from build123d import *

# Parameters (mm, degrees)
SKETCH2_W           = 110
SKETCH2_H           = 83
SKETCH2_W_2         = 10
SKETCH2_H_2         = 40
BOSS_EXTRUDE1_DEPTH = 9
SKETCH4_W           = 103
SKETCH4_H           = 77.5
CUT_EXTRUDE1_DEPTH  = 6


with BuildPart() as part:
    # Sketch2 → Boss-Extrude1 (new body)
    with BuildSketch(Plane(origin=(0, 0, 0), x_dir=(1, 0, 0), z_dir=(0, 1, 0))):
        Rectangle(SKETCH2_W, SKETCH2_H)
        with Locations((46, 0)):
            Rectangle(SKETCH2_W_2, SKETCH2_H_2, mode=Mode.SUBTRACT)
    extrude(amount=BOSS_EXTRUDE1_DEPTH)

    # Sketch4 → Cut-Extrude1 (cut)
    with BuildSketch(Plane(origin=(0, 9, 0), x_dir=(1, 0, 0), z_dir=(0, 1, 0))):
        Rectangle(SKETCH4_W, SKETCH4_H)
    extrude(amount=-CUT_EXTRUDE1_DEPTH, mode=Mode.SUBTRACT)


solid = part.part
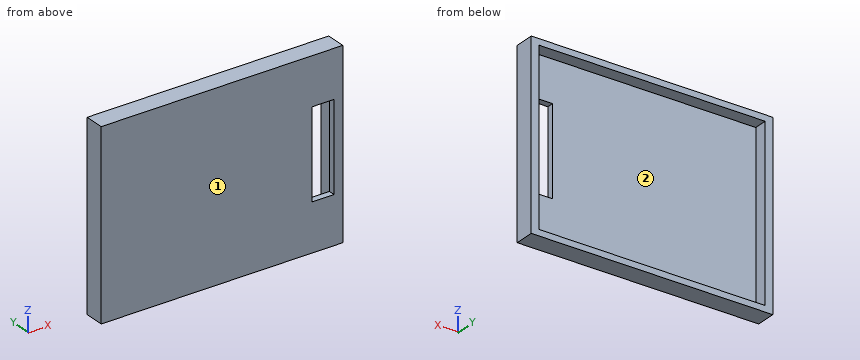
Geometry: final body of the model. Coordinates: model frame, mm. Face numbers are marked on the shaded views. Give positions to 0.01 mm unless a question says otherwise; leave off trailing zeros. Write each loop counter-clockwise with the first axis right and the second up, starting at its lowest first coordinate (ties: lowest second). Pieces come first, ordered by that corner, then holes. Notation, with made-up numbers: (57.25, 72) - (84.25, 72) arc R27 ccw to (84.25, 101) - close; hole circle Ø9 at (58, 5). An arc over 180 degrees is marked (long way). Return JSON: item names as keys, results as strings. Group by question number.
1) Section A-A on z = 17.5. Return the cut outline in (x, y), plus the area to 3 significant figures.
2) Line query: line 1 (Z direction, x = -25, y = 3.25); line 2 (X direction, y = 7.5, z = 32.5); line 3 (Z direction, x = 50, y = 1). Output: solid intervals per line, ascending.
3) Section B-B on z = -22.5. Return the cut outline in (x, y).
4) Mould query, pull axis X, two halves, no side actions, for the marked faces 1 and 2. Classes: released by +X, released by -X, zero draft, split by the parting line, or undercut.
5) Section C-C on y = 5.5. Return the cut outline in (x, z).
6) Section D-D on x = 10. Return the cut outline in (y, z).
7) First-contact query: P1, Ø1, axis at x = -6.5, z = -30, coming from the -Y side; P2, Ø23, axis at x = 19.5, z = -6.5, coming from the +Y side. Flat tips, straight axial feed; report the tip coordinate or a pass-through.
Filled in:
{
 "1": {"outline": "(-55, 0) - (41, 0) - (41, 3) - (-51.5, 3) - (-51.5, 9) - (-55, 9) - close; (51, 0) - (55, 0) - (55, 9) - (51.5, 9) - (51.5, 3) - (51, 3) - close", "area": "342 mm^2"},
 "2": {"line 1": "z = -41.5 to -38.75, 38.75 to 41.5", "line 2": "x = -55 to -51.5, 51.5 to 55", "line 3": "z = -41.5 to -20, 20 to 41.5"},
 "3": {"outline": "(-55, 0) - (55, 0) - (55, 9) - (51.5, 9) - (51.5, 3) - (-51.5, 3) - (-51.5, 9) - (-55, 9) - close"},
 "4": {"face 1": "zero draft", "face 2": "undercut"},
 "5": {"outline": "(-55, -41.5) - (55, -41.5) - (55, 41.5) - (-55, 41.5) - close; hole (-51.5, -38.75) - (51.5, -38.75) - (51.5, 38.75) - (-51.5, 38.75) - close"},
 "6": {"outline": "(0, -41.5) - (9, -41.5) - (9, -38.75) - (3, -38.75) - (3, 38.75) - (9, 38.75) - (9, 41.5) - (0, 41.5) - close"},
 "7": {"P1": "stops at y = 0", "P2": "stops at y = 3"}
}
